from build123d import *

# Parameters (mm, degrees)
F0_W     = 304.8
F0_H     = 190.5
F0_W_2   = 38.1
F1_DEPTH = 38.1
F2_DEPTH = 38.1
F3_DEPTH = 38.1
F4_DEPTH = 38.1
F0_W_3   = 1447.8
F0_H_2   = 838.2
F5_DEPTH = 76.2
F6_DEPTH = 76.2
F7_DEPTH = 76.2


with BuildPart() as f1:
    # F0 (on Front) → F1 (new body)
    with BuildSketch(Plane.XZ):
        with Locations((-190.5, -133.35)):
            Rectangle(F0_W, F0_H)
        with Locations((-361.95, -133.35)):
            Rectangle(F0_W_2, F0_H)
        Polygon((-381, -228.6), (-381, -38.1), (-1066.8, -38.1), (-1067.900241926, -228.6), align=None)
        Polygon((-1067.900241926, -228.6), (-1066.8, -38.1), (-1104.9, -38.1), (-1104.9, -228.6), align=None)
        with Locations((-1257.3, -133.35)):
            Rectangle(F0_W, F0_H)
    extrude(amount=F1_DEPTH)

    # F0 (on Front) → F2 (join)
    with BuildSketch(Plane.XZ):
        Polygon((-38.1, -427.021741867), (-38.1, -228.6), (-342.9, -228.6), (-342.9, -425.2613547854), align=None)
        Polygon((-342.9, -425.2613547854), (-342.9, -228.6), (-381, -228.6), (-381, -425.0413064002), align=None)
        Polygon((-381, -425.0413064002), (-381, -228.6), (-1067.900241926, -228.6), (-1069.0118481718, -421.0676608311), align=None)
        Polygon((-1069.0118481718, -421.0676608311), (-1067.900241926, -228.6), (-1104.9, -228.6), (-1104.9, -420.8603870816), align=None)
        Polygon((-1104.9, -420.8603870816), (-1104.9, -228.6), (-1409.7, -228.6), (-1409.7, -419.1), align=None)
    extrude(amount=F2_DEPTH)

    # F0 (on Front) → F3 (join)
    with BuildSketch(Plane.XZ):
        Polygon((-38.1, -609.6), (-38.1, -427.021741867), (-342.9, -425.2613547854), (-342.9, -607.8396129184), align=None)
        Polygon((-342.9, -607.8396129184), (-342.9, -425.2613547854), (-381, -425.0413064002), (-381, -607.6195645333), align=None)
        Polygon((-381, -607.6195645333), (-381, -425.0413064002), (-1069.0118481718, -421.0676608311), (-1070.0663025227, -603.6398289122), align=None)
        Polygon((-1070.0663025227, -603.6398289122), (-1069.0118481718, -421.0676608311), (-1104.9, -420.8603870816), (-1104.9, -603.4386452146), align=None)
        Polygon((-1104.9, -603.4386452146), (-1104.9, -420.8603870816), (-1409.7, -419.1), (-1409.7, -601.678258133), align=None)
    extrude(amount=F3_DEPTH)

    # F0 (on Front) → F4 (join)
    with BuildSketch(Plane.XZ):
        Polygon((-38.1, -800.1), (-38.1, -609.6), (-342.9, -607.8396129184), (-342.9, -800.1), align=None)
        Polygon((-342.9, -800.1), (-342.9, -607.8396129184), (-381, -607.6195645333), (-381, -800.1), align=None)
        Polygon((-381, -800.1), (-381, -607.6195645333), (-1070.0663025227, -603.6398289122), (-1071.2009677039, -800.1), align=None)
        Polygon((-1071.2009677039, -800.1), (-1070.0663025227, -603.6398289122), (-1104.9, -603.4386452146), (-1104.9, -800.1), align=None)
        Polygon((-1104.9, -800.1), (-1104.9, -603.4386452146), (-1409.7, -601.678258133), (-1409.7, -800.1), align=None)
    extrude(amount=F4_DEPTH)

    # F0 (on Front) → F5 (join)
    with BuildSketch(Plane.XZ):
        with Locations((-723.9, -419.1)):
            Rectangle(F0_W_3, F0_H_2)
        Polygon((-342.9, -38.1), (-38.1, -38.1), (-38.1, -228.6), (-38.1, -427.021741867), (-38.1, -609.6), (-38.1, -800.1), (-342.9, -800.1), (-381, -800.1), (-1071.2009677039, -800.1), (-1104.9, -800.1), (-1409.7, -800.1), (-1409.7, -601.678258133), (-1409.7, -419.1), (-1409.7, -228.6), (-1409.7, -38.1), (-1104.9, -38.1), (-1066.8, -38.1), (-381, -38.1), align=None, mode=Mode.SUBTRACT)
    extrude(amount=F5_DEPTH)

    # F0 (on Front) → F6 (join)
    with BuildSketch(Plane.XZ):
        Polygon((-1067.900241926, -228.6), (-1066.8, -38.1), (-1104.9, -38.1), (-1104.9, -228.6), align=None)
        Polygon((-1069.0118481718, -421.0676608311), (-1067.900241926, -228.6), (-1104.9, -228.6), (-1104.9, -420.8603870816), align=None)
        Polygon((-1070.0663025227, -603.6398289122), (-1069.0118481718, -421.0676608311), (-1104.9, -420.8603870816), (-1104.9, -603.4386452146), align=None)
        Polygon((-1071.2009677039, -800.1), (-1070.0663025227, -603.6398289122), (-1104.9, -603.4386452146), (-1104.9, -800.1), align=None)
    extrude(amount=F6_DEPTH)

    # F0 (on Front) → F7 (join)
    with BuildSketch(Plane.XZ):
        with Locations((-361.95, -133.35)):
            Rectangle(F0_W_2, F0_H)
        Polygon((-342.9, -425.2613547854), (-342.9, -228.6), (-381, -228.6), (-381, -425.0413064002), align=None)
        Polygon((-342.9, -607.8396129184), (-342.9, -425.2613547854), (-381, -425.0413064002), (-381, -607.6195645333), align=None)
        Polygon((-342.9, -800.1), (-342.9, -607.8396129184), (-381, -607.6195645333), (-381, -800.1), align=None)
    extrude(amount=F7_DEPTH)


solid = f1.part
For this review, take the finished solid that the model builds, in its own axes (mm). A direction names the side the tool comes from. Round coordinates to 2 decimals unless told otherwise and drop trailing zeros. Loops run counter-clockwise (first coordinate to the right, second up) from the corner with the lowest first, then second, coordinate; pieces in that order, holes last. Notation, with made-up numbers: (-31, -22.5) - (-21, -22.5) arc R25 ccw to (-21, 2.5) - close; hole circle Ø4 at (-17, 66.5). An arc over 180 degrees is marked (long way). Use one line per item in the form item = value.
1) Wall thickness on probe 1 along Z at (x, y) = (-1355.5, -45); probe 2 along X at (y, z) = (-39.5, -401.5); probe 3 along X at (y, z) = (-45.5, -347): over which ranges is each line inside the solid? List them lowest first.
Solutions:
probe_1 = -838.2 to -800.1, -38.1 to 0
probe_2 = -1447.8 to -1409.7, -1104.9 to -1068.9, -381 to -342.9, -38.1 to 0
probe_3 = -1447.8 to -1409.7, -1104.9 to -1068.58, -381 to -342.9, -38.1 to 0
2) Tool access review of faces 1 (the face through (-1103, -76.2, -386)), 2 (the face through (-1255, -57, -800.1)): name each direction out of +Z, -Z, +X, -X, +Y, -Y from which nothing blocks a thin tool from reaching the whole face with its end or side.
Solutions:
face_1 = +Z, -Z, +X, -X, -Y
face_2 = -Y
3) We need section C-C on z = -768. Write out the cut boundary in (x, y).
Solutions:
outline = (-1447.8, -76.2) - (-1409.7, -76.2) - (-1409.7, -38.1) - (-1104.9, -38.1) - (-1104.9, -76.2) - (-1071.02, -76.2) - (-1071.02, -38.1) - (-381, -38.1) - (-381, -76.2) - (-342.9, -76.2) - (-342.9, -38.1) - (-38.1, -38.1) - (-38.1, -76.2) - (0, -76.2) - (0, 0) - (-1447.8, 0) - close
4) We need section A-A on y = -50. Write out the cut boundary in (x, z).
Solutions:
outline = (-1447.8, -838.2) - (0, -838.2) - (0, 0) - (-1447.8, 0) - close; hole (-1409.7, -800.1) - (-1104.9, -800.1) - (-1104.9, -38.1) - (-1409.7, -38.1) - close; hole (-1071.2, -800.1) - (-381, -800.1) - (-381, -38.1) - (-1066.8, -38.1) - close; hole (-342.9, -800.1) - (-38.1, -800.1) - (-38.1, -38.1) - (-342.9, -38.1) - close
5) We need section D-D on z = -362. Write out the cut boundary in (x, y), then the cut area to 3 significant figures.
Solutions:
outline = (-1447.8, -76.2) - (-1409.7, -76.2) - (-1409.7, -38.1) - (-1104.9, -38.1) - (-1104.9, -76.2) - (-1068.67, -76.2) - (-1068.67, -38.1) - (-381, -38.1) - (-381, -76.2) - (-342.9, -76.2) - (-342.9, -38.1) - (-38.1, -38.1) - (-38.1, -76.2) - (0, -76.2) - (0, 0) - (-1447.8, 0) - close
area = 60,900 mm2
6) Clearance check with a flat-ended pin moving along its axis: P1, Ø8, axis at x = -891, z = -524.5, coming from the -Y side. State where the tip first meets the part, or that it passes through.
Solutions:
P1 = -38.1
7) We need section B-B on x = -628. Write out the cut boundary in (y, z), then the cut area to 3 significant figures.
Solutions:
outline = (-76.2, -838.2) - (0, -838.2) - (0, 0) - (-76.2, 0) - (-76.2, -38.1) - (-38.1, -38.1) - (-38.1, -800.1) - (-76.2, -800.1) - close
area = 34,800 mm2
8) Mouldability with a two-part tool opening along X and no side actions: class faces 3 (the face through (-729, -57, -38.1)), 4 (the face through (-734, -38, 0)), 5 (the face through (0, -38, -425)), 6 (the face through (-721, -57, -800.1)) as pulls with the +X half, pulls with the -X half, needs draft (parallel to the pull), parting line crosses it, or undercut.
Solutions:
face_3 = undercut
face_4 = needs draft
face_5 = pulls with the +X half
face_6 = undercut
